Part print with two shaded views. Sizes in mm from the minimum x, y, z corner. Round coordinates to 2 decimals unless told otherwise and drop trailing zeros. Loops run counter-clockwise (first coordinate to the right, second up) from the corner with the lowest first, then second, coordinate; pieces in that order, holes last. Notation, with made-up numbers: M 73.25,88 L 90.25,88 A18 ccw 90.25,93 Z; hole C 31,68 d5. An arc over 180 degrees is marked long. Answer as CSV lines item,"result". Start each with the question number.
Item 1: Band-saw the part on C-C (x = 159.5). Give the cut face in (y, z), and give its area (3 significant figures).
Item 2: Drop flat-ended pins along their axis: pin 1 Ø8 at (y, z) = (5, 213) entering from -X (1 decimal); pin 2 Ø4.5 at (x, z) = (382.89, 382.89) entering from -Y; pin 3 Ø3 at (y, z) = (9.5, 438) entering from -X (1 decimal); pin 4 Ø7.5 at (y, z) = (15.5, 432) entering from +X. Give the stop position or say it passes through.
Item 3: Band-saw the part on D-D (y = 3.75). Count the separate pieces of the cut face and the enclosed holes in it, and give its area (3 significant figures).
Item 4: Band-saw the part on B-B (z = 245). Give the cut face in (x, y), and give its area (3 significant figures).
Item 5: Wall check: line 1 (Z direction, x = 245, y = 11.5); line 2 (Z direction, x = 210, y = 17.75); line 3 (X direction, y = 12.75, z = 251). Give the ranges that are in metal, low to high.
Item 6: Band-saw the part on A-A (x = 245). Give the cut face in (y, z).
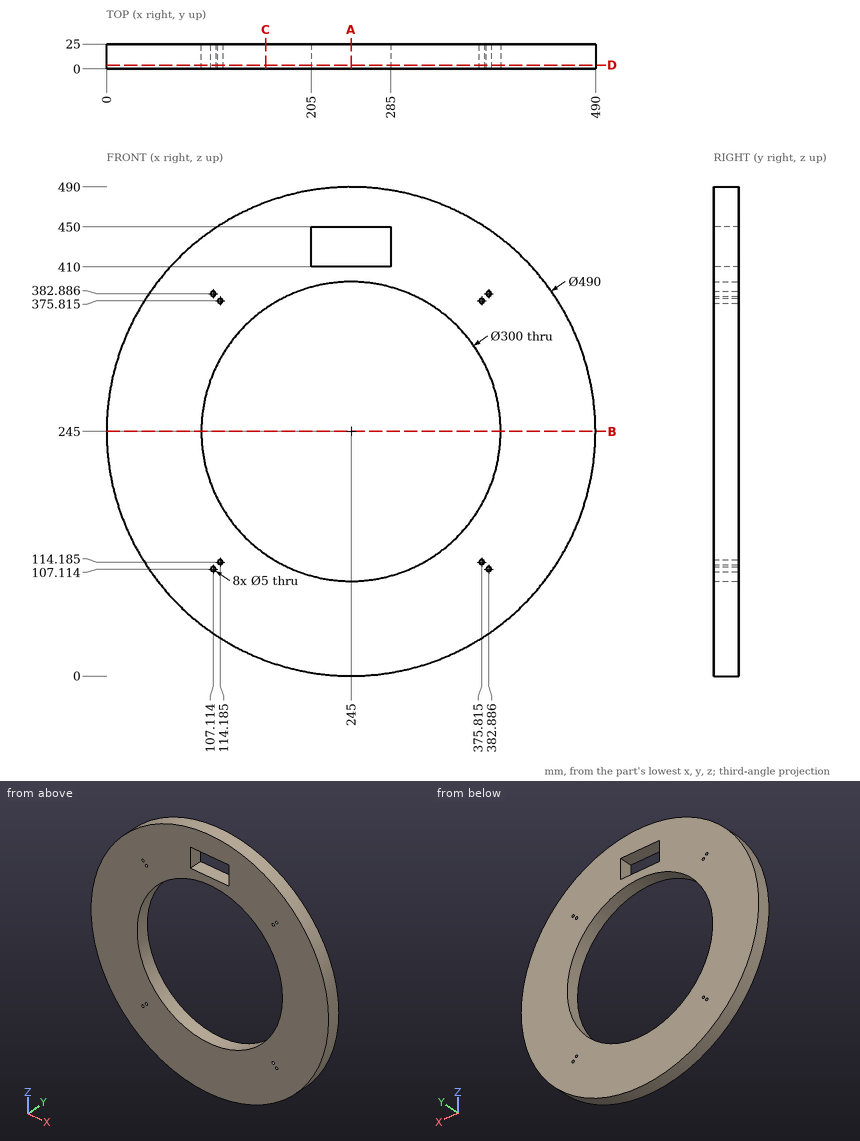
Answer block:
1,outline,"M 0,15.4 L 25,15.4 L 25,121.75 L 0,121.75 Z; M 0,368.25 L 25,368.25 L 25,474.6 L 0,474.6 Z"
1,area,"5,320 mm^2"
2,pin 1,"stops at x = 1.6"
2,pin 2,"passes through"
2,pin 3,"stops at x = 92.2"
2,pin 4,"stops at x = 407.62"
3,separate pieces,"1"
3,enclosed holes,"10"
3,area,"115,000 mm^2"
4,outline,"M 0,0 L 95,0 L 95,25 L 0,25 Z; M 395,0 L 490,0 L 490,25 L 395,25 Z"
4,area,"4,750 mm^2"
5,line 1,"z = 0 to 95, 395 to 410, 450 to 490"
5,line 2,"z = 2.51 to 99.14, 390.86 to 410, 450 to 487.49"
5,line 3,"x = 0.07 to 95.12, 394.88 to 489.93"
6,outline,"M 0,0 L 25,0 L 25,95 L 0,95 Z; M 0,395 L 25,395 L 25,410 L 0,410 Z; M 0,450 L 25,450 L 25,490 L 0,490 Z"
